from build123d import *

# Parameters (mm, degrees)
BOSS_EXTRUDE1_DEPTH = 3.175
FILLET1_R           = 1.5875


with BuildPart() as part:
    # Sketch1 → Boss-Extrude1 (new, symmetric)
    with BuildSketch(Plane.XY):
        with BuildLine():
            Line((-1.27, 10.670267616), (-1.27, 12.7))
            ThreePointArc((-1.27, 12.7), (-1.084012806, 13.149012806), (-0.635, 13.335))
            Line((-0.635, 13.335), (0.635, 13.335))
            ThreePointArc((0.635, 13.335), (1.084012806, 13.149012806), (1.27, 12.7))
            Line((1.27, 12.7), (1.27, 10.670267616))
            ThreePointArc((1.27, 10.670267616), (1.583306834, 9.753271395), (2.392223502, 9.219701281))
            Line((2.392223502, 9.219701281), (2.538124316, 9.180607276))
            ThreePointArc((2.538124316, 9.180607276), (3.505451757, 9.238234215), (4.235281545, 9.875722821))
            Line((4.235281545, 9.875722821), (5.250147737, 11.633522628))
            ThreePointArc((5.250147737, 11.633522628), (5.635723775, 11.929385528), (6.117573869, 11.865948759))
            Line((6.117573869, 11.865948759), (7.217426131, 11.230948759))
            ThreePointArc((7.217426131, 11.230948759), (7.513289031, 10.845372722), (7.449852263, 10.363522628))
            Line((7.449852263, 10.363522628), (6.434986071, 8.605722821))
            ThreePointArc((6.434986071, 8.605722821), (6.247819637, 7.654927381), (6.681576965, 6.788383774))
            Line((6.681576965, 6.788383774), (6.788383774, 6.681576965))
            ThreePointArc((6.788383774, 6.681576965), (7.654927381, 6.247819637), (8.605722821, 6.434986071))
            Line((8.605722821, 6.434986071), (10.363522628, 7.449852263))
            ThreePointArc((10.363522628, 7.449852263), (10.845372722, 7.513289031), (11.230948759, 7.217426131))
            Line((11.230948759, 7.217426131), (11.865948759, 6.117573869))
            ThreePointArc((11.865948759, 6.117573869), (11.929385528, 5.635723775), (11.633522628, 5.250147737))
            Line((11.633522628, 5.250147737), (9.875722821, 4.235281545))
            ThreePointArc((9.875722821, 4.235281545), (9.238234215, 3.505451757), (9.180607276, 2.538124316))
            Line((9.180607276, 2.538124316), (9.219701281, 2.392223502))
            ThreePointArc((9.219701281, 2.392223502), (9.753271395, 1.583306834), (10.670267616, 1.27))
            Line((10.670267616, 1.27), (12.7, 1.27))
            ThreePointArc((12.7, 1.27), (13.149012806, 1.084012806), (13.335, 0.635))
            Line((13.335, 0.635), (13.335, -0.635))
            ThreePointArc((13.335, -0.635), (13.149012806, -1.084012806), (12.7, -1.27))
            Line((12.7, -1.27), (10.670267616, -1.27))
            ThreePointArc((10.670267616, -1.27), (9.753271395, -1.583306834), (9.219701281, -2.392223502))
            Line((9.219701281, -2.392223502), (9.180607276, -2.538124316))
            ThreePointArc((9.180607276, -2.538124316), (9.238234215, -3.505451757), (9.875722821, -4.235281545))
            Line((9.875722821, -4.235281545), (11.633522628, -5.250147737))
            ThreePointArc((11.633522628, -5.250147737), (11.929385528, -5.635723775), (11.865948759, -6.117573869))
            Line((11.865948759, -6.117573869), (11.230948759, -7.217426131))
            ThreePointArc((11.230948759, -7.217426131), (10.845372722, -7.513289031), (10.363522628, -7.449852263))
            Line((10.363522628, -7.449852263), (8.605722821, -6.434986071))
            ThreePointArc((8.605722821, -6.434986071), (7.654927381, -6.247819637), (6.788383774, -6.681576965))
            Line((6.788383774, -6.681576965), (6.681576965, -6.788383774))
            ThreePointArc((6.681576965, -6.788383774), (6.247819637, -7.654927381), (6.434986071, -8.605722821))
            Line((6.434986071, -8.605722821), (7.449852263, -10.363522628))
            ThreePointArc((7.449852263, -10.363522628), (7.513289031, -10.845372722), (7.217426131, -11.230948759))
            Line((7.217426131, -11.230948759), (6.117573869, -11.865948759))
            ThreePointArc((6.117573869, -11.865948759), (5.635723775, -11.929385528), (5.250147737, -11.633522628))
            Line((5.250147737, -11.633522628), (4.235281545, -9.875722821))
            ThreePointArc((4.235281545, -9.875722821), (3.505451757, -9.238234215), (2.538124316, -9.180607276))
            Line((2.538124316, -9.180607276), (2.392223502, -9.219701281))
            ThreePointArc((2.392223502, -9.219701281), (1.583306834, -9.753271395), (1.27, -10.670267616))
            Line((1.27, -10.670267616), (1.27, -12.7))
            ThreePointArc((1.27, -12.7), (1.084012806, -13.149012806), (0.635, -13.335))
            Line((0.635, -13.335), (-0.635, -13.335))
            ThreePointArc((-0.635, -13.335), (-1.084012806, -13.149012806), (-1.27, -12.7))
            Line((-1.27, -12.7), (-1.27, -10.670267616))
            ThreePointArc((-1.27, -10.670267616), (-1.583306834, -9.753271395), (-2.392223502, -9.219701281))
            Line((-2.392223502, -9.219701281), (-2.538124316, -9.180607276))
            ThreePointArc((-2.538124316, -9.180607276), (-3.505451757, -9.238234215), (-4.235281545, -9.875722821))
            Line((-4.235281545, -9.875722821), (-5.250147737, -11.633522628))
            ThreePointArc((-5.250147737, -11.633522628), (-5.635723775, -11.929385528), (-6.117573869, -11.865948759))
            Line((-6.117573869, -11.865948759), (-7.217426131, -11.230948759))
            ThreePointArc((-7.217426131, -11.230948759), (-7.513289031, -10.845372722), (-7.449852263, -10.363522628))
            Line((-7.449852263, -10.363522628), (-6.434986071, -8.605722821))
            ThreePointArc((-6.434986071, -8.605722821), (-6.247819637, -7.654927381), (-6.681576965, -6.788383774))
            Line((-6.681576965, -6.788383774), (-6.788383774, -6.681576965))
            ThreePointArc((-6.788383774, -6.681576965), (-7.654927381, -6.247819637), (-8.605722821, -6.434986071))
            Line((-8.605722821, -6.434986071), (-10.363522628, -7.449852263))
            ThreePointArc((-10.363522628, -7.449852263), (-10.845372722, -7.513289031), (-11.230948759, -7.217426131))
            Line((-11.230948759, -7.217426131), (-11.865948759, -6.117573869))
            ThreePointArc((-11.865948759, -6.117573869), (-11.929385528, -5.635723775), (-11.633522628, -5.250147737))
            Line((-11.633522628, -5.250147737), (-9.875722821, -4.235281545))
            ThreePointArc((-9.875722821, -4.235281545), (-9.238234215, -3.505451757), (-9.180607276, -2.538124316))
            Line((-9.180607276, -2.538124316), (-9.219701281, -2.392223502))
            ThreePointArc((-9.219701281, -2.392223502), (-9.753271395, -1.583306834), (-10.670267616, -1.27))
            Line((-10.670267616, -1.27), (-12.7, -1.27))
            ThreePointArc((-12.7, -1.27), (-13.149012806, -1.084012806), (-13.335, -0.635))
            Line((-13.335, -0.635), (-13.335, 0.635))
            ThreePointArc((-13.335, 0.635), (-13.149012806, 1.084012806), (-12.7, 1.27))
            Line((-12.7, 1.27), (-10.670267616, 1.27))
            ThreePointArc((-10.670267616, 1.27), (-9.753271395, 1.583306834), (-9.219701281, 2.392223502))
            Line((-9.219701281, 2.392223502), (-9.180607276, 2.538124316))
            ThreePointArc((-9.180607276, 2.538124316), (-9.238234215, 3.505451757), (-9.875722821, 4.235281545))
            Line((-9.875722821, 4.235281545), (-11.633522628, 5.250147737))
            ThreePointArc((-11.633522628, 5.250147737), (-11.929385528, 5.635723775), (-11.865948759, 6.117573869))
            Line((-11.865948759, 6.117573869), (-11.230948759, 7.217426131))
            ThreePointArc((-11.230948759, 7.217426131), (-10.845372722, 7.513289031), (-10.363522628, 7.449852263))
            Line((-10.363522628, 7.449852263), (-8.605722821, 6.434986071))
            ThreePointArc((-8.605722821, 6.434986071), (-7.654927381, 6.247819637), (-6.788383774, 6.681576965))
            Line((-6.788383774, 6.681576965), (-6.681576965, 6.788383774))
            ThreePointArc((-6.681576965, 6.788383774), (-6.247819637, 7.654927381), (-6.434986071, 8.605722821))
            Line((-6.434986071, 8.605722821), (-7.449852263, 10.363522628))
            ThreePointArc((-7.449852263, 10.363522628), (-7.513289031, 10.845372722), (-7.217426131, 11.230948759))
            Line((-7.217426131, 11.230948759), (-6.117573869, 11.865948759))
            ThreePointArc((-6.117573869, 11.865948759), (-5.635723775, 11.929385528), (-5.250147737, 11.633522628))
            Line((-5.250147737, 11.633522628), (-4.235281545, 9.875722821))
            ThreePointArc((-4.235281545, 9.875722821), (-3.505451757, 9.238234215), (-2.538124316, 9.180607276))
            Line((-2.538124316, 9.180607276), (-2.392223502, 9.219701281))
            ThreePointArc((-2.392223502, 9.219701281), (-1.583306834, 9.753271395), (-1.27, 10.670267616))
        make_face()
        Polygon((-3.666174209, 6.35), (-7.332348419, 0), (-3.666174209, -6.35), (3.666174209, -6.35), (7.332348419, 0), (3.666174209, 6.35), align=None, mode=Mode.SUBTRACT)
    extrude(amount=BOSS_EXTRUDE1_DEPTH, both=True)

    # Fillet1
    fillet1_edges = [part.edges().sort_by_distance(p)[0] for p in [
        (-3.666174209, 6.35, 0),
        (-7.332348419, 0, 0),
        (-3.666174209, -6.35, 0),
        (3.666174209, -6.35, 0),
        (7.332348419, 0, 0),
        (3.666174209, 6.35, 0),
    ]]
    fillet(fillet1_edges, radius=FILLET1_R)


solid = part.part
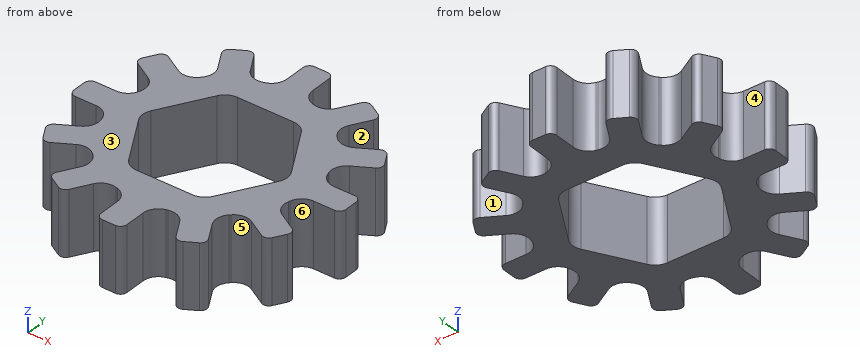
The model under review builds one solid part; all positions refer to its coordinate system, in mm. Face numbers are marked on the shaded views. A direction names the side the tool comes from. Round coordinates to 2 decimals unless told otherwise and drop trailing zeros. Write each loop counter-clockwise with the first axis right and the second up, starting at its lowest first coordinate (ties: lowest second). Pieces come first, ordered by that corner, then holes. Notation, with made-up numbers: M 5.5,66.5 L 21.5,66.5 A25 cw 21.5,80.5 Z; hole C -23,60 d8. An arc over 180 degrees is marked long. Use a Markdown table: item, result. Add a question column.
Q1. We need section C-C, the plane x = -8. State the section outline as (y, z) points (3 decimals).
Q2. To check wall thickness, follow line 1 (Y direction, x = 9.5, z = 0.75); line 2 (Y direction, x = -0.5, z = 2) (3 decimals). State the ranges of each line that lie inside material, in increasing order.
Q3. We need section A-A, the plane y = 0. State the section outline as (x, z) points (3 decimals).
Q4. Insertion check: pin 1 (3 mm diameter, centred on x = 3, y = 1, fed in from -Z); pin 2 (3 mm diameter, centred on x = 2.5, z = -1, fed in from -Y); pin 3 (2 mm diameter, centred on y = 12, z = 0.5, fed in from +X); pin 4 (0.6 mm diameter, centred on y = -12, z = -0.5, fed in from +X) (3 decimals). Each pin has a flat end and moves straight along its axis. Give the tip position at first contact, or say it passes through.
Q5. Machinability: for the marked faces 4, 5 and 6, which of the approach directions +Z, -Z, +X, -X, +Y, -Y give a long, thin tool a straight path to every point of the face, cutting with its end or side? Answer none if there is none.
Q6. We need section B-B, the plane x = -1.75. State the section outline as (y, z) points (3 decimals), plus the area to 3 significant figures.
Q7. The part is to be moulded in two halves that separate along Y. For the marked faces 1, 2 and 3, say which applies: pulls with the +Y half, pulls with the -Y half, needs draft (parallel to the pull), parting line crosses it, or undercut.
Findings below:
| question | item | result |
|---|---|---|
| 1 | outline | M -6.241,-3.175 L 6.241,-3.175 L 6.241,3.175 L -6.241,3.175 Z |
| 2 | line 1 | y = -6.95 to -3.93, -1.83 to 1.83, 3.93 to 6.95 |
| 2 | line 2 | y = -13.335 to -6.35, 6.35 to 13.335 |
| 3 | outline | M -13.335,-3.175 L -7.087,-3.175 L -7.087,3.175 L -13.335,3.175 Z; M 7.087,-3.175 L 13.335,-3.175 L 13.335,3.175 L 7.087,3.175 Z |
| 4 | pin 1 | passes through |
| 4 | pin 2 | stops at y = -13.22 |
| 4 | pin 3 | stops at x = 7.45 |
| 4 | pin 4 | stops at x = 6.405 |
| 5 | face 4 | +Z, -Z, -X |
| 5 | face 5 | +Z, -Z |
| 5 | face 6 | +Z, -Z, +X |
| 6 | outline | M -9.571,-3.175 L -6.35,-3.175 L -6.35,3.175 L -9.571,3.175 Z; M 6.35,-3.175 L 9.571,-3.175 L 9.571,3.175 L 6.35,3.175 Z |
| 6 | area | 40.9 mm² |
| 7 | face 1 | pulls with the +Y half |
| 7 | face 2 | undercut |
| 7 | face 3 | needs draft |
